Verification items for this drawing (mm, ordinates from the low corner). Coordinates: 2 decimals unless noted, no trailing zeros. Loops run counter-clockwise (first coordinate to the right, second up) from the corner with the lowest first, then second, coordinate; pieces in that order, holes last. Notation, with made-up numbers: (-38, 14.5) -> (-32, 14.5) arc R9 ccw to (-32, 22.5) -> close; hole circle Ø9 at (31, 56.25). An arc over 180 degrees is marked (long way). Write item = value, one per line.
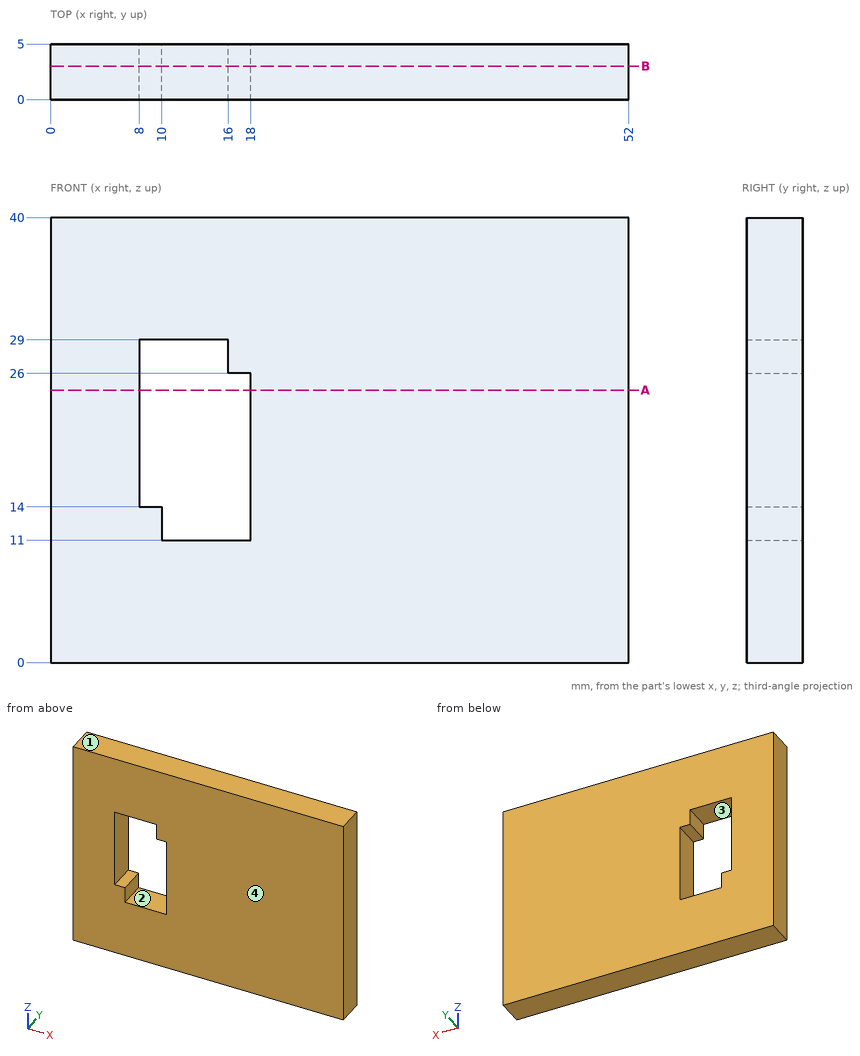
1) Material ranges on line 1 (X direction, y = 2.2, z = 17.5); line 2 (Z direction, x = 8.5, y = 3.6); line 3 (X direction, y = 3, z = 28.5), recorded low to high.
Ans:
line_1 = 0 to 8, 18 to 52
line_2 = 0 to 14, 29 to 40
line_3 = 0 to 8, 16 to 52
2) Sectioned sample at A-A, the plane z = 24.5. Record the cut outline in (x, y), plus the area to 3 significant figures.
Ans:
outline = (0, 0) -> (8, 0) -> (8, 5) -> (0, 5) -> close; (18, 0) -> (52, 0) -> (52, 5) -> (18, 5) -> close
area = 210 mm2
3) Release check for a two-part mould opening along Z. For the marked faces 1, 2, 3 and 4 record: pulls with the +Z half, pulls with the -Z half, needs draft (parallel to the pull), parting line crosses it, or undercut.
Ans:
face_1 = pulls with the +Z half
face_2 = undercut
face_3 = undercut
face_4 = needs draft
4) Sectioned sample at B-B, the plane y = 3. Record the cut outline in (x, z), plus the area to 3 significant figures.
Ans:
outline = (0, 0) -> (52, 0) -> (52, 40) -> (0, 40) -> close; hole (8, 14) -> (10, 14) -> (10, 11) -> (18, 11) -> (18, 26) -> (16, 26) -> (16, 29) -> (8, 29) -> close
area = 1,910 mm2
